For this review, take the finished solid that the model builds, in its own axes (mm). Round coordinates to 2 decimals unless told otherwise and drop trailing zeros. Write each loop counter-clockwise with the first axis right and the second up, starting at its lowest first coordinate (ties: lowest second). Pieces come first, ordered by that corner, then holes. Notation, with made-up numbers: M -15,43 L 8,43 A16 ccw 8,66 Z; hole C -20.75,43.25 d6. An arc over 180 degrees is marked long. Use one line per item in the form item = value. Start each with the question number.
Item 1: Add section A-A (y = 144.5). State the section outline as (x, z) points, and give its area (3 significant figures).
Item 2: For line 1 (Y direction, x = 65, z = 2.05); line 2 (Y direction, x = -65, z = 1.15); line 3 (X direction, y = -26.5, z = 0.9), list the stretches that pass through material, from the lowest coordinate up. Write a range as [from, to].
Item 3: Add section C-C (x = 45.5). State the section outline as (y, z) points, and give its area (3 significant figures).
Item 4: Add section B-B (z = 2.3). Count the separate pieces of the cut face and the enclosed holes in it, and give its area (3 significant figures).
Item 5: For P1, Ø5, axis at x = -65, y = 200.9, coming from the +Z side; P2, Ø3, axis at x = -39.5, y = 57, coming from the -Z side, all flat-tipped, find the tip position at first contact; note any pin that passes through.
Item 6: Add section D-D (y = 193). State the section outline as (x, z) points.
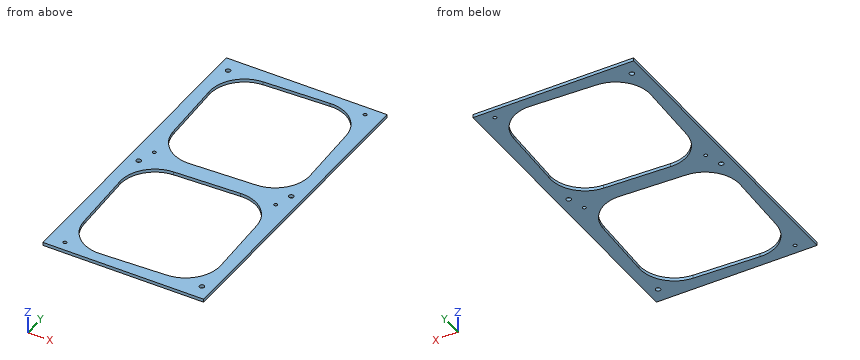
Autodesk Inventor part; units mm, degrees
ref_plane "YZ Plane" through (0, 0, 0) normal (1, 0, 0) x (0, 1, 0)
ref_plane "XZ Plane" through (0, 0, 0) normal (0, 1, 0) x (-1, 0, 0)
ref_plane "XY Plane" through (0, 0, 0) normal (0, 0, 1) x (1, 0, 0)
sketch "スケッチ1" plane through (0, 0, 0) normal (0, 0, 1) x (1, 0, 0)
  line L0 (-75, -215) -> (75, -215)
  line L1 (75, -215) -> (75, 215)
  line L2 (75, 215) -> (-75, 215)
  line L3 (-75, 215) -> (-75, -215)
  line L4 (-75, -215) -> (75, 215) construction
  line L5 (75, -215) -> (-75, 215) construction
  line L6 (-65, -215) -> (-65, 215) construction
  line L7 (-65, 59.8957) -> (59.8957, 65) construction
  line L8 (59.8957, 65) -> (65, -59.8957) construction
  line L9 (65, -59.8957) -> (-59.8957, -65) construction
  line L10 (-59.8957, -65) -> (-65, 59.8957) construction
  line L11 (-65, 59.8957) -> (65, -59.8957) construction
  line L12 (59.8957, 65) -> (-59.8957, -65) construction
  circle A0 centre (-65, 59.8957) radius 2.25
  line L13 (-67.0832, -72.8) -> (72.8, -67.0832) construction
  line L14 (72.8, -67.0832) -> (67.0832, 72.8) construction
  line L15 (67.0832, 72.8) -> (-72.8, 67.0832) construction
  line L16 (-72.8, 67.0832) -> (-67.0832, -72.8) construction
  line L17 (-67.0832, -72.8) -> (67.0832, 72.8) construction
  line L18 (72.8, -67.0832) -> (-72.8, 67.0832) construction
  line L19 (0, 0) -> (0, 70.0584) construction
  circle A1 centre (65, -59.8957) radius 2.25
  circle A2 centre (59.8957, 65) radius 1.6
  circle A3 centre (-59.8957, -65) radius 1.6
  line L20 (-63.6933, 27.9224) -> (-61.2024, -33.0267)
  line L21 (-27.9224, -63.6933) -> (33.0267, -61.2024)
  line L22 (63.6933, -27.9224) -> (61.2024, 33.0267)
  line L23 (27.9224, 63.6933) -> (-33.0267, 61.2024)
  line L24 (-62.4479, -2.5521) -> (62.4479, 2.5521) construction
  arc A4 (-33.0267, 61.2024) -> (-63.6933, 27.9224) centre (-31.72, 29.2291) ccw
  arc A5 (61.2024, 33.0267) -> (27.9224, 63.6933) centre (29.2291, 31.72) ccw
  arc A6 (33.0267, -61.2024) -> (63.6933, -27.9224) centre (31.72, -29.2291) ccw
  arc A7 (-61.2024, -33.0267) -> (-27.9224, -63.6933) centre (-29.2291, -31.72) ccw
  circle A8 centre (-65, -81.1043) radius 2.25
  circle A9 centre (-59.8957, -206) radius 1.6
  circle A10 centre (65, -200.8957) radius 2.25
  circle A11 centre (59.8957, -76) radius 1.6
  arc A12 (61.2024, -107.9733) -> (27.9224, -77.3067) centre (29.2291, -109.28) ccw
  line L25 (27.9224, -77.3067) -> (-33.0267, -79.7976)
  arc A13 (-33.0267, -79.7976) -> (-63.6933, -113.0776) centre (-31.72, -111.7709) ccw
  line L26 (-63.6933, -113.0776) -> (-61.2024, -174.0267)
  arc A14 (-61.2024, -174.0267) -> (-27.9224, -204.6933) centre (-29.2291, -172.72) ccw
  line L27 (-27.9224, -204.6933) -> (33.0267, -202.2024)
  arc A15 (33.0267, -202.2024) -> (63.6933, -168.9224) centre (31.72, -170.2291) ccw
  line L28 (63.6933, -168.9224) -> (61.2024, -107.9733)
  circle A16 centre (-65, 200.8957) radius 2.25
  circle A17 centre (-59.8957, 76) radius 1.6
  circle A18 centre (65, 81.1043) radius 2.25
  circle A19 centre (59.8957, 206) radius 1.6
  arc A20 (61.2024, 174.0267) -> (27.9224, 204.6933) centre (29.2291, 172.72) ccw
  line L29 (27.9224, 204.6933) -> (-33.0267, 202.2024)
  arc A21 (-33.0267, 202.2024) -> (-63.6933, 168.9224) centre (-31.72, 170.2291) ccw
  line L30 (-63.6933, 168.9224) -> (-61.2024, 107.9733)
  arc A22 (-61.2024, 107.9733) -> (-27.9224, 77.3067) centre (-29.2291, 109.28) ccw
  line L31 (-27.9224, 77.3067) -> (33.0267, 79.7976)
  arc A23 (33.0267, 79.7976) -> (63.6933, 113.0776) centre (31.72, 111.7709) ccw
  line L32 (63.6933, 113.0776) -> (61.2024, 174.0267)
  circle A24 centre (-65, 59.8957) radius 2.25
  circle A25 centre (-59.8957, -65) radius 1.6
  circle A26 centre (65, -59.8957) radius 2.25
  circle A27 centre (59.8957, 65) radius 1.6
  arc A28 (61.2024, 33.0267) -> (27.9224, 63.6933) centre (29.2291, 31.72) ccw
  line L33 (27.9224, 63.6933) -> (-33.0267, 61.2024)
  arc A29 (-33.0267, 61.2024) -> (-63.6933, 27.9224) centre (-31.72, 29.2291) ccw
  line L34 (-63.6933, 27.9224) -> (-61.2024, -33.0267)
  arc A30 (-61.2024, -33.0267) -> (-27.9224, -63.6933) centre (-29.2291, -31.72) ccw
  line L35 (-27.9224, -63.6933) -> (33.0267, -61.2024)
  arc A31 (33.0267, -61.2024) -> (63.6933, -27.9224) centre (31.72, -29.2291) ccw
  line L36 (63.6933, -27.9224) -> (61.2024, 33.0267)
  point P0 (-65, 59.8957)
  point P1 (59.8957, 65)
  point P2 (-65, -81.1043)
  point P3 (59.8957, -76)
  point P4 (-62.4479, -143.5521)
  point P5 (62.4479, -138.4479)
  point P6 (-65, 200.8957)
  point P7 (59.8957, 206)
  point P8 (-62.4479, 138.4479)
  point P9 (62.4479, 143.5521)
  point P10 (-65, 59.8957)
  point P11 (59.8957, 65)
  dimension "d0" = 150
  dimension "d1" = 430
  dimension "d3" = 65
  dimension "d4" = 125
  dimension "d7" = 4.5
  dimension "d8" = 140
  dimension "d9" = 70.0584
  dimension "d10" = 3.2
  dimension "d24" = 125
  dimension "d25" = 32
  dimension "d28" = 141
  dimension "d31" = 141
extrude "押し出し1" add sketch "スケッチ1" along normal blind 3 contours L3 L2 L1 L0 | A8 | A9 | A10 | A11
sketch "スケッチ4" plane through (0, 0, 3) normal (0, 0, 1) x (1, 0, 0)
  line L0 (-75, -215) -> (75, -215) construction
  line L1 (-75, -215) -> (75, -215)
  line L2 (75, -215) -> (75, -74)
  line L3 (75, -74) -> (-75, -74)
  line L4 (-75, -74) -> (-75, -215)
  point P0 (0, 0)
  dimension "d43" = 141
extrude "押し出し3" cut sketch "スケッチ4" against normal through all
properties part number "top_140mm" material "アルミニウム 6061"
Calculated:
q1.outline = M -75,0 L -62.7,0 L -62.7,3 L -75,3 Z; M 62.41,0 L 75,0 L 75,3 L 62.41,3 Z
q1.area = 74.7 mm^2
q2.line_1 = [-74, -62.15], [-57.65, 78.85], [83.35, 215]
q2.line_2 = [-74, 57.65], [62.15, 198.65], [203.15, 215]
q2.line_3 = [-75, -61.47], [63.64, 75]
q3.outline = M -74,0 L -58.11,0 L -58.11,3 L -74,3 Z; M 59.27,0 L 82.89,0 L 82.89,3 L 59.27,3 Z; M 200.27,0 L 215,0 L 215,3 L 200.27,3 Z
q3.area = 163 mm^2
q4.separate_pieces = 1
q4.enclosed_holes = 10
q4.area = 13,800 mm^2
q5.P1 = 3
q5.P2 = through
q6.outline = M -75,0 L -54.2,0 L -54.2,3 L -75,3 Z; M 53.98,0 L 75,0 L 75,3 L 53.98,3 Z
